```python
from build123d import *

# Parameters (mm, degrees)
F0_W     = 25.4
F0_H     = 50.8
F1_DEPTH = 50.8
F2_W     = 35.56
F2_H     = 35.56
F3_DEPTH = 12.7
F4_W     = 17.088712
F4_H     = 6.858
F5_DEPTH = 7.62
F6_W     = 17.0942
F6_H     = 6.858
F7_DEPTH = 7.62


with BuildPart() as f1:
    # F0 (on Front) → F1 (new body)
    with BuildSketch(Plane.XZ):
        with Locations((12.7, 25.4)):
            Rectangle(F0_W, F0_H)
    extrude(amount=F1_DEPTH)

    # F2 (on face) → F3 (cut)
    with BuildSketch(Plane.YZ.offset(25.4)):
        with Locations((-25.4, 25.4)):
            Rectangle(F2_W, F2_H)
    extrude(amount=-F3_DEPTH, mode=Mode.SUBTRACT)

    # F4 (on face) → F5 (cut)
    with BuildSketch(Plane.XZ.offset(50.8)):
        with Locations((16.855644, 39.116)):
            Rectangle(F4_W, F4_H)
        with Locations((16.855644, 25.4)):
            Rectangle(F4_W, F4_H)
        with Locations((16.855644, 11.684)):
            Rectangle(F4_W, F4_H)
    extrude(amount=-F5_DEPTH, mode=Mode.SUBTRACT)

    # F6 (on face) → F7 (cut)
    with BuildSketch(Plane(origin=(0, 0, 0), x_dir=(-1, 0, 0), z_dir=(0, 1, 0))):
        with Locations((-16.8529, 39.116)):
            Rectangle(F6_W, F6_H)
        with Locations((-16.8529, 25.4)):
            Rectangle(F6_W, F6_H)
        with Locations((-16.8529, 11.684)):
            Rectangle(F6_W, F6_H)
    extrude(amount=-F7_DEPTH, mode=Mode.SUBTRACT)


solid = f1.part
```
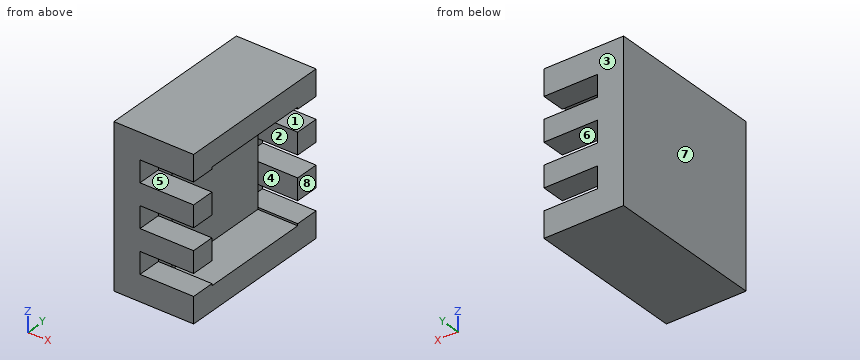
Source: CAD feature listing. Evaluate the final solid. Frame: model axes, mm. Face numbers are marked on the shaded views. A direction names the side the tool comes from. Give positions to 0.01 mm unless a question says otherwise; leave off trailing zeros. Loops run counter-clockwise (first coordinate to the right, second up) from the corner with the lowest first, then second, coordinate; pieces in that order, holes last. Notation, with made-up numbers: (58.5, 0.5) - (107.5, 0.5) arc R15 ccw to (107.5, 27.5) - close; hole circle Ø1 at (40.25, 34.25). An arc over 180 degrees is marked (long way). Use CSV: the item, a comma, the result in double quotes. Start each with the question number.
1. Section D-D (x = 9.25). Output: boundary loops of the cut face in (y, z) (3 decimals), then the cut area to 3 significant figures.
2. Draft query along Y for the marked faces 1, 2 and 3. Return one class per face: +Y half, -Y half, draft (parallel to the pull), parting line (faces both ways), or undercut.
3. Reachability of the marked faces 4, 5, 6, 7 and 8 from +Z, -Z, +X, -X, +Y, -Y: full face, straight path, thin tool, end or side. Return the list, or none.
4. Pin query (flat end, axial travel): pin 1 (3.5 mm diameter, centred on y = -2, z = 27, fed in from +X); pin 2 (5 mm diameter, centred on y = -40, z = 15, fed in from +X); pin 3 (3.5 mm diameter, centred on x = 11, z = 25, fed in from -Y). Return the tip coordinate at first contact, or that it passes through.
5. Section A-A (x = 19). Count the separate pieces of the cut face and the enclosed holes in it, then the cut area to 3 significant figures.
6. Ray query, L1, parallel to Z at x = 20, y = -47 (3 decimals); L2, parallel to Y at x = 22.25, z = 29; L3, parallel to Z at x = 20.5, y = -25. Return the intervals inside material, ascending.
7. Section C-C (y = -29.5). Output: boundary loops of the cut face in (x, z).
8. Section B-B (z = 17.5). Output: boundary loops of the cut face in (x, y).
Response:
1,outline,"(-50.8, 0) - (0, 0) - (0, 8.255) - (-7.62, 8.255) - (-7.62, 15.113) - (0, 15.113) - (0, 21.971) - (-7.62, 21.971) - (-7.62, 28.829) - (0, 28.829) - (0, 35.687) - (-7.62, 35.687) - (-7.62, 42.545) - (0, 42.545) - (0, 50.8) - (-50.8, 50.8) - (-50.8, 42.545) - (-43.18, 42.545) - (-43.18, 35.687) - (-50.8, 35.687) - (-50.8, 28.829) - (-43.18, 28.829) - (-43.18, 21.971) - (-50.8, 21.971) - (-50.8, 15.113) - (-43.18, 15.113) - (-43.18, 8.255) - (-50.8, 8.255) - close"
1,area,"2,270 mm²"
2,face 1,"draft"
2,face 2,"undercut"
2,face 3,"+Y half"
3,face 4,"+X"
3,face 5,"+X, -Y"
3,face 6,"+X, +Y"
3,face 7,"+Z, -Z, -X, +Y, -Y"
3,face 8,"+Z, -Z, +X, +Y, -Y"
4,pin 1,"x = 8.31"
4,pin 2,"x = 12.7"
4,pin 3,"y = -43.18"
5,separate pieces,"6"
5,enclosed holes,"0"
5,area,"1,000 mm²"
6,L1,"0 to 8.255, 15.113 to 21.971, 28.829 to 35.687, 42.545 to 50.8"
6,L2,"-50.8 to -43.18, -7.62 to 0"
6,L3,"0 to 7.62, 43.18 to 50.8"
7,outline,"(0, 0) - (25.4, 0) - (25.4, 7.62) - (12.7, 7.62) - (12.7, 43.18) - (25.4, 43.18) - (25.4, 50.8) - (0, 50.8) - close"
8,outline,"(0, -50.8) - (25.4, -50.8) - (25.4, -43.18) - (12.7, -43.18) - (12.7, -7.62) - (25.4, -7.62) - (25.4, 0) - (0, 0) - close"
